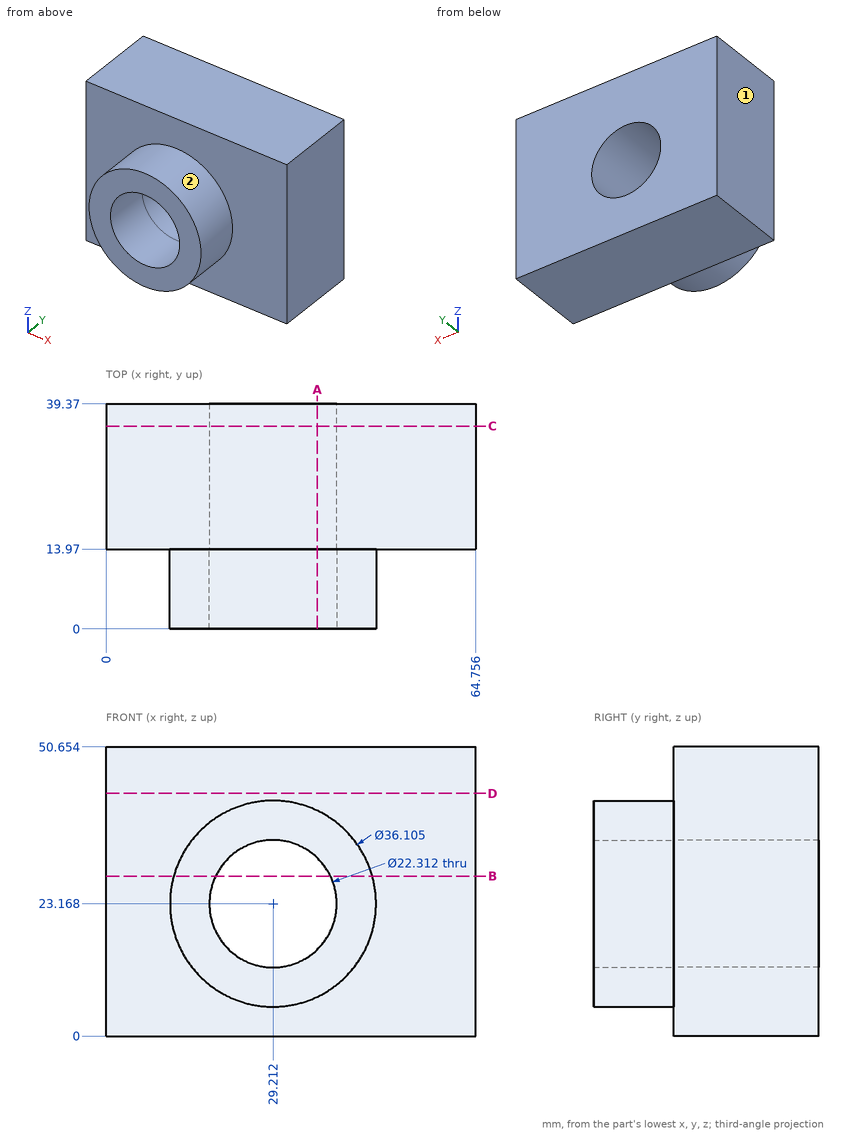
Geometry: see drawing. Coordinates: mm, zero at the bounding-box minimum. A direction names the side the tool comes from. Give positions to 0.01 mm unless a question says otherwise; leave off trailing zeros. Loops run counter-clockwise (first coordinate to the right, second up) from the corner with the lowest first, then second, coordinate; pieces in that order, holes last. Notation, with made-up numbers: (30.5, 33) -> (82.5, 33) arc R22 cw to (82.5, 61) -> close; hole circle Ø8 at (57.25, -36.5). An arc over 180 degrees is marked (long way). Answer as a JSON object with one key per item and string values. Group by question number.
Item 1: Reachability of the marked faces 1 and 2 from +Z, -Z, +X, -X, +Y, -Y: full face, straight path, thin tool, end or side. Return the list, or none.
Item 2: Pin query (flat end, axial travel): P1, Ø1, axis at y = 11, z = 12, coming from the +X side (1 decimal); P2, Ø12, axis at x = 36, y = 18, coming from the -Z side. Return the tip coordinate at first contact, or that it passes through.
Item 3: Cut plane C-C, the plane y = 35.5. Return the cut outline in (x, z) (1 decimal), and give its area (3 significant figures).
Item 4: Cut plane A-A, the plane x = 37. Return the cut outline in (y, z) (1 decimal).
Item 5: Line query: probe 1 along Z at (x, y) = (29, 31) (1 decimal); probe 2 along Y at (x, z) = (18, 45); probe 3 along Z at (x, y) = (32, 5) (1 decimal). Output: solid intervals per line, ascending.
Item 6: Cut plane D-D, the plane z = 42.5. Return the cut outline in (x, y), and give its area (3 significant figures).
Item 7: Cut plane B-B, the plane z = 28. Return the cut outline in (x, y).
Checks:
{
 "1": {"face 1": "+Z, -Z, -X, +Y, -Y", "face 2": "-Y"},
 "2": {"P1": "stops at x = 43.8", "P2": "stops at z = 0"},
 "3": {"outline": "(0, 0) -> (64.8, 0) -> (64.8, 50.7) -> (0, 50.7) -> close; hole circle Ø22.3 at (29.2, 23.2)", "area": "2,890 mm²"},
 "4": {"outline": "(0, 6.9) -> (14, 6.9) -> (14, 0) -> (39.4, 0) -> (39.4, 15.2) -> (0, 15.2) -> close; (0, 31.2) -> (39.4, 31.2) -> (39.4, 50.7) -> (14, 50.7) -> (14, 39.5) -> (0, 39.5) -> close"},
 "5": {"probe 1": "z = 0 to 12, 34.3 to 50.7", "probe 2": "y = 13.97 to 39.37", "probe 3": "z = 5.3 to 12.4, 34 to 41"},
 "6": {"outline": "(0, 13.97) -> (64.76, 13.97) -> (64.76, 39.37) -> (0, 39.37) -> close", "area": "1,640 mm²"},
 "7": {"outline": "(0, 13.97) -> (11.82, 13.97) -> (11.82, 0) -> (19.16, 0) -> (19.16, 39.37) -> (0, 39.37) -> close; (39.27, 0) -> (46.61, 0) -> (46.61, 13.97) -> (64.76, 13.97) -> (64.76, 39.37) -> (39.27, 39.37) -> close"}
}
